Design review of the part built by this model. Coordinates are the model's own, in mm. Coordinates: 2 decimals unless noted, no trailing zeros. Write each loop counter-clockwise with the first axis right and the second up, starting at its lowest first coordinate (ties: lowest second). Pieces come first, ordered by that corner, then holes.
Q1. Insertion check: pin 1 (1.5 mm diameter, centred on x = 3.5, z = 1, fed in from +Y); pin 2 (1.5 mm diameter, centred on x = 5.5, z = 2, fed in from +Y). Each pin has a flat end and moves straight along its axis. Give the tip position at first contact, or say it passes through.
Q2. For probe 1 along Y at (x, z) = (10.75, 2.4); probe 2 along Y at (x, z) = (-10, 1.3); probe 3 along Y at (x, z) = (-12.5, 1.35), list the stretches that pass through material, from the lowest coordinate up.
Q3. Take a section at A-A (z = 1.5). Give the boundary of the cut face in (x, y).
Q4. Take a section at D-D (y = 2). Give the boundary of the cut face in (x, z).
Q5. Take a section at B-B (y = 10.5). Give the boundary of the cut face in (x, z), and give its area (3 significant figures).
Q6. Mouldability with a two-part tool opening along Y and no side actions: class faces 1 (the flat face through (-5.755, -11.412, 1.479)), 2 (the flat face through (0, 0, 3)), 3 (the cylindrical face through (11, 10.32, 1.48)) as pulls with the +Y half, pulls with the -Y half, needs draft (parallel to the pull), parting line crosses it, or undercut.
Q7. Take a section at C-C (x = -6). Give the boundary of the cut face in (y, z).
```python
from build123d import *

# Parameters (mm, degrees)
SKETCH1_R           = 1.05
BOSS_EXTRUDE1_DEPTH = 3


with BuildPart() as part:
    # Sketch1 → Boss-Extrude1 (new body)
    with BuildSketch(Plane.XY):
        with BuildLine():
            Line((2.752454122, 8.409308372), (8.843145751, 14.5))
            Line((8.843145751, 14.5), (10, 14.5))
            ThreePointArc((10, 14.5), (13.181980515, 13.181980515), (14.5, 10))
            Line((14.5, 10), (14.5, 8.843145751))
            Line((14.5, 8.843145751), (8.409308372, 2.752454122))
            ThreePointArc((8.409308372, 2.752454122), (6.256695253, -6.256695253), (-2.752454122, -8.409308372))
            Line((-2.752454122, -8.409308372), (-8.843145751, -14.5))
            Line((-8.843145751, -14.5), (-10, -14.5))
            ThreePointArc((-10, -14.5), (-13.181980515, -13.181980515), (-14.5, -10))
            Line((-14.5, -10), (-14.5, -8.843145751))
            Line((-14.5, -8.843145751), (-8.409308372, -2.752454122))
            ThreePointArc((-8.409308372, -2.752454122), (-6.256695253, 6.256695253), (2.752454122, 8.409308372))
        make_face()
        with Locations((10, 10)):
            Circle(SKETCH1_R, mode=Mode.SUBTRACT)
        with Locations((-10, -10)):
            Circle(SKETCH1_R, mode=Mode.SUBTRACT)
    extrude(amount=BOSS_EXTRUDE1_DEPTH)


solid = part.part
```
Response:
1. pin 1: stops at y = 9.91
1. pin 2: stops at y = 11.91
2. probe 1: y = 5.09 to 9.27, 10.73 to 14.44
2. probe 2: y = -14.5 to -11.05, -8.95 to -4.34
2. probe 3: y = -13.74 to -6.84
3. outline: (-14.5, -10) arc R4.5 ccw to (-10, -14.5) - (-8.84, -14.5) - (-2.75, -8.41) arc R8.85 ccw to (8.41, 2.75) - (14.5, 8.84) - (14.5, 10) arc R4.5 ccw to (10, 14.5) - (8.84, 14.5) - (2.75, 8.41) arc R8.85 ccw to (-8.41, -2.75) - (-14.5, -8.84) - close; hole circle Ø2.1 at (-10, -10); hole circle Ø2.1 at (10, 10)
4. outline: (-8.62, 0) - (8.62, 0) - (8.62, 3) - (-8.62, 3) - close
5. outline: (4.84, 0) - (9.08, 0) - (9.08, 3) - (4.84, 3) - close; (10.92, 0) - (14.47, 0) - (14.47, 3) - (10.92, 3) - close
5. area: 23.3 mm2
6. face 1: pulls with the -Y half
6. face 2: needs draft
6. face 3: undercut
7. outline: (-11.66, 0) - (6.5, 0) - (6.5, 3) - (-11.66, 3) - close
